Here's how the part is built. I have some questions about the finished solid (model axes, mm). A direction names the side the tool comes from. Round coordinates to 2 decimals unless told otherwise and drop trailing zeros. Order: outer loops, then holes, each group sorted by start corner. A loop starts at its lowest first (then second) coordinate and runs counter-clockwise, first axis right, second up. Notation, with made-up numbers: (-12, 24) - (-4, 24) arc R5 ccw to (-4, 30) - close; hole circle Ø3 at (70, 3). An arc over 180 degrees is marked (long way). Answer as a JSON object with one key per item and string values.
```python
from build123d import *

# Parameters (mm, degrees)
F1_DEPTH = 6.35
F2_R     = 5.08
F3_DEPTH = 25.4
F4_DEPTH = 3.81
F5_DEPTH = 5.08


with BuildPart() as f1:
    # F0 (on Top) → F1 (new body, symmetric)
    with BuildSketch(Plane.XY):
        with BuildLine():
            ThreePointArc((-8.150841, 5.930474), (-9.027019, 6.212621), (-9.893435, 6.523457))
            Line((-9.893435, 6.523457), (-11.928295, 1.434566))
            ThreePointArc((-11.928295, 1.434566), (0.246561, -0.797492), (12.378132, 1.65897))
            Line((12.378132, 1.65897), (9.853429, 6.523457))
            ThreePointArc((9.853429, 6.523457), (8.987013, 6.212621), (8.110835, 5.930474))
            ThreePointArc((8.110835, 5.930474), (-0.020003, 4.722101), (-8.150841, 5.930474))
        make_face()
    extrude(amount=F1_DEPTH, both=True)

    # F2 (on Front) → F3 (join)
    with BuildSketch(Plane.XZ):
        Circle(F2_R)
    extrude(amount=F3_DEPTH)

    # F0 (on Top) → F4 (join, symmetric)
    with BuildSketch(Plane.XY):
        with BuildLine():
            Line((-4.892698, 53.244065), (-9.893435, 6.523457))
            ThreePointArc((-9.893435, 6.523457), (-9.027019, 6.212621), (-8.150841, 5.930474))
            Line((-8.150841, 5.930474), (-4.892698, 49.243495))
            Line((-4.892698, 49.243495), (0, 53.244065))
            Line((0, 53.244065), (4.8927, 50.282495))
            Line((4.8927, 50.282495), (8.110835, 5.930474))
            ThreePointArc((8.110835, 5.930474), (8.987013, 6.212621), (9.853429, 6.523457))
            Line((9.853429, 6.523457), (4.8927, 53.244065))
            Line((4.8927, 53.244065), (0, 57.244636))
            Line((0, 57.244636), (-4.892698, 53.244065))
        make_face()
    extrude(amount=F4_DEPTH, both=True)

    # F0 (on Top) → F5 (join, symmetric)
    with BuildSketch(Plane.XY):
        with BuildLine():
            Line((-4.892698, 49.243495), (-8.150841, 5.930474))
            ThreePointArc((-8.150841, 5.930474), (-0.020003, 4.722101), (8.110835, 5.930474))
            Line((8.110835, 5.930474), (4.8927, 50.282495))
            Line((4.8927, 50.282495), (0, 53.244065))
            Line((0, 53.244065), (-4.892698, 49.243495))
        make_face()
    extrude(amount=F5_DEPTH, both=True)


solid = f1.part
```
1. Imagine slicing it at D-D (x = -3.75). List the corners of the cut face in (y, z) for me, plus the area to 3 significant figures.
Responses:
{"outline": "(-25.4, -3.43) - (-0.59, -3.43) - (-0.59, -6.35) - (4.97, -6.35) - (4.97, -5.08) - (50.18, -5.08) - (50.18, -3.81) - (54.18, -3.81) - (54.18, 3.81) - (50.18, 3.81) - (50.18, 5.08) - (4.97, 5.08) - (4.97, 6.35) - (-0.59, 6.35) - (-0.59, 3.43) - (-25.4, 3.43) - close", "area": "730 mm2"}
2. For faces 1 (the face through (-7, 32, 3.81)), 2 (the face through (-7, 32, -3.81)), 3 (the face through (2.481, 51.743, 4.454)), 4 (the face through (2.481, 51.743, -4.436)), which set-ups out of +Z, -Z, +X, -X, +Y, -Y let a thin tool reach every point of the face, with its end or its side?
Responses:
{"face 1": "+Z, +Y", "face 2": "-Z, +Y", "face 3": "+Z, +X, +Y", "face 4": "-Z, +X, +Y"}
3. If I drill on L1, parallel to Z at x = 7.5, y = 26; L2, parallel to Z at x = -5, y = 42.5; L3, parallel to X at y = 37.5, z = 0, over which ranges is the centre line in solid material (lowest first)? Write a range as [from, to].
Responses:
{"L1": "[-3.81, 3.81]", "L2": "[-5.08, 5.08]", "L3": "[-6.58, 6.56]"}
4. For P1, Ø6, axis at x = 0, y = 30.5, coming from the +Z side; P2, Ø6, axis at x = 0, y = 36.5, coming from the -Z side; P3, Ø6, axis at y = 47.5, z = 1, coming from the -X side, each with a flat end and sliding along its axis, tell me the tip position at first contact or that it passes through.
Responses:
{"P1": "z = 5.08", "P2": "z = -5.08", "P3": "x = -5.83"}
5. Imagine slicing it at A-A (x = 4). List the corners of the cut face in (y, z) for me.
Responses:
{"outline": "(-25.4, -3.13) - (-0.55, -3.13) - (-0.55, -6.35) - (5.01, -6.35) - (5.01, -5.08) - (50.82, -5.08) - (50.82, -3.81) - (53.97, -3.81) - (53.97, 3.81) - (50.82, 3.81) - (50.82, 5.08) - (5.01, 5.08) - (5.01, 6.35) - (-0.55, 6.35) - (-0.55, 3.13) - (-25.4, 3.13) - close"}
6. Imagine slicing it at C-C (z = 0). List the corners of the cut face in (x, y) for me.
Responses:
{"outline": "(-11.93, 1.43) arc R32.68 ccw to (-5.08, -0.41) - (-5.08, -25.4) - (5.08, -25.4) - (5.08, -0.39) arc R32.68 ccw to (12.38, 1.66) - (9.85, 6.52) - (4.89, 53.24) - (0, 57.24) - (-4.89, 53.24) - (-9.89, 6.52) - close"}
7. Imagine slicing it at B-B (y = 39). List the corners of the cut face in (x, z) for me.
Responses:
{"outline": "(-6.42, -3.81) - (-5.66, -3.81) - (-5.66, -5.08) - (5.71, -5.08) - (5.71, -3.81) - (6.41, -3.81) - (6.41, 3.81) - (5.71, 3.81) - (5.71, 5.08) - (-5.66, 5.08) - (-5.66, 3.81) - (-6.42, 3.81) - close"}
